```python
from build123d import *

# Parameters (mm, degrees)
SKETCH_1_R      = 10
EXTRUDE_1_DEPTH = 10


with BuildPart() as part:
    # 스케치1 → 보스-돌출1 (new body)
    with BuildSketch(Plane(origin=(0, 0, 0), x_dir=(1, 0, 0), z_dir=(0, 1, 0))):
        with Locations(Location((0, 0, 0), (0, 0, 270))):
            Circle(SKETCH_1_R)
        with BuildLine():
            ThreePointArc((5, 0), (-2.942731468, -4.042317591), (-1.536132603, 4.758182071))
            Line((-1.536132603, 4.758182071), (-1.536132603, 6.856766437))
            Line((-1.536132603, 6.856766437), (1.428204445, 6.856766437))
            Line((1.428204445, 6.856766437), (1.428204445, 4.791683636))
            ThreePointArc((1.428204445, 4.791683636), (4.0088042, 2.98822504), (5, 0))
        make_face(mode=Mode.SUBTRACT)
    extrude(amount=EXTRUDE_1_DEPTH)


solid = part.part
```
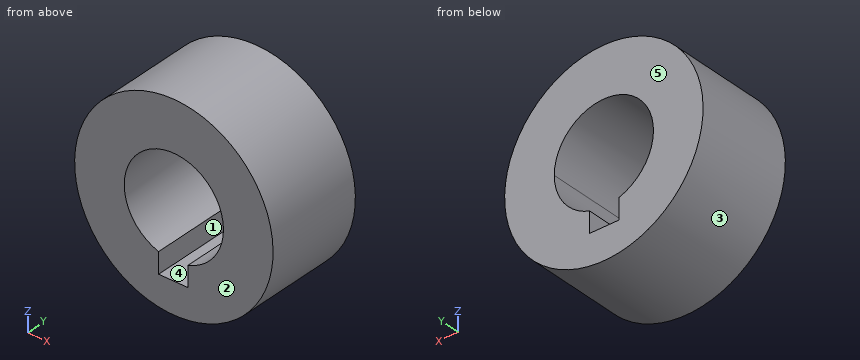
Input: part model. Units: mm. Frame: model coordinates. Face numbers are marked on the shaded views. A direction names the side the tool comes from. Round coordinates to 2 decimals unless told otherwise and drop trailing zeros. Loops run counter-clockwise (first coordinate to the right, second up) from the corner with the lowest first, then second, coordinate; pieces in that order, holes last. Notation, with made-up numbers: (31, -20.5) - (77, -20.5) arc R16 ccw to (77, -1.5) - close; hole circle Ø10 at (-35.5, 82). An arc over 180 degrees is marked (long way). One line per item, written item: value. Start each with the question number.
(1) Ray query, line 1 (X direction, y = 2.5, z = 0); line 2 (X direction, y = 1.25, z = 3.25); line 3 (Z direction, x = -2.25, y = 9). Return the intervals inside material, ascending. Write a range as [from, to].
(2) Draft query along Z for the marked faces 1, 2 and 3. Return one class per face: +Z half, -Z half, draft (parallel to the pull), parting line (faces both ways), or undercut.
(3) Access query for the marked faces 4 and 5. Directions: +Z, -Z, +X, -X, +Y, -Y. A direction counts if a zero-diameter tool reaches every point of the face in a straight line with its end or side. Return the directions, or none.
(4) Section D-D, the plane x = -7. Return loops of the section in (y, z), plus the area to 3 significant figures.
(5) Contact query for flat-ended pins moving along their axis: P1, Ø0.6, axis at y = 3, z = -5.5, coming from the -X side; P2, Ø1.7, axis at y = 2.5, z = -5.5, coming from the +X side; P3, Ø4, axis at y = 2, z = -2.5, coming from the -X side. Output: stop coordinate, or through.
(6) Section B-B, the plane z = -6. Return loops of the section in (x, y), plus the area to 3 significant figures.
(7) Section A-A, the plane x = 0. Return loops of the section in (y, z).
(8) Section C-C, the plane y = 5.5. Return loops of the section in (x, z), plus the area to 3 significant figures.
Results below:
1. line 1: [-10, -5], [5, 10]
1. line 2: [-9.46, -3.8], [3.8, 9.46]
1. line 3: [-9.74, -4.47], [4.47, 9.74]
2. face 1: undercut
2. face 2: draft
2. face 3: parting line
3. face 4: +Y, -Y
3. face 5: +Z, -Z, +X, -X, +Y
4. outline: (0, -7.14) - (10, -7.14) - (10, 7.14) - (0, 7.14) - close
4. area: 143 mm^2
5. P1: x = -8.54
5. P2: x = 8.85
5. P3: x = -9.99
6. outline: (-8, 0) - (-1.54, 0) - (-1.54, 10) - (-8, 10) - close; (1.43, 0) - (8, 0) - (8, 10) - (1.43, 10) - close
6. area: 130 mm^2
7. outline: (0, -10) - (10, -10) - (10, -6.86) - (0, -6.86) - close; (0, 5) - (10, 5) - (10, 10) - (0, 10) - close
8. outline: circle Ø20 at (0, 0); hole (-1.54, -6.86) - (1.43, -6.86) - (1.43, -4.79) arc R5 ccw (long way) to (-1.54, -4.76) - close
8. area: 230 mm^2
